Answer from the drawing. Dimensions are ordinates in mm from the lowest x, y and z of the part. A direction names the side the tool comes from. Give positions to 0.01 mm unless a question says otherwise; leave off trailing zeros. Write each loop counter-clockwise with the first axis right and the second up, starting at its lowest first coordinate (ties: lowest second). Pieces come first, ordered by that corner, then holes.
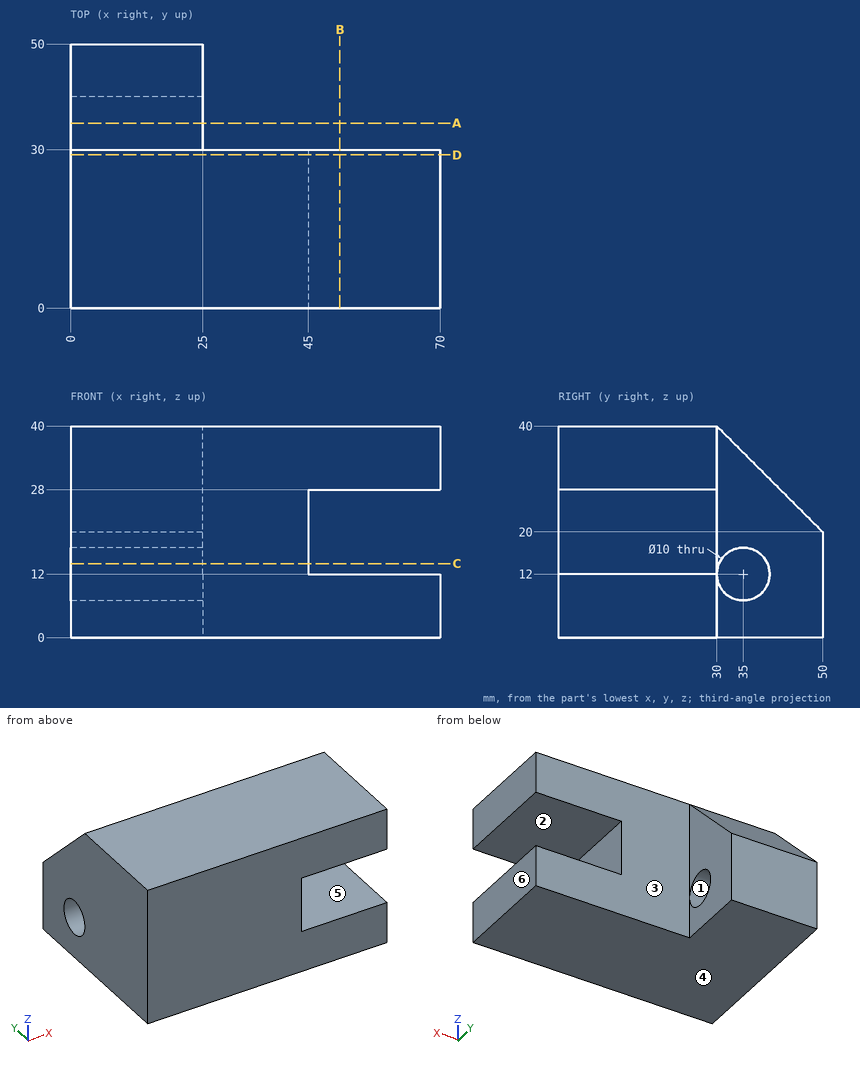
Item 1: Determine the mould class of the marked faces 4, 5 and 6 for opening direction Z: pulls with the +Z half, pulls with the -Z half, needs draft (parallel to the pull), parting line crosses it, or undercut.
Conclusion:
face 4: pulls with the -Z half
face 5: undercut
face 6: needs draft
Item 2: Which of the six approach directions +Z, -Z, +X, -X, +Y, -Y give full straight-line access (tool end or side, diameter ignored) to the marked faces 1, 2 and 3?
Conclusion:
face 1: +X, -X
face 2: +X, +Y, -Y
face 3: +Z, -Z, +X, +Y
Item 3: A cutting plane is placed at D-D, the plane y = 29. Give the vertices of the cut face in (x, z), plus the area to 3 significant figures.
Conclusion:
outline: (0, 0) - (70, 0) - (70, 12) - (45, 12) - (45, 28) - (70, 28) - (70, 40) - (0, 40) - close
area: 2,400 mm2
Item 4: Each of these flat-tipped pins is pushed along its axis until it touches: P1, Ø10, axis at y = 36.5, z = 25.5, coming from the +X side; P2, Ø5, axis at y = 8, z = 23.5, coming from the +X side; P3, Ø5, axis at x = 23.5, z = 35, coming from the +Y side. Where does it stop, or does it pass through?
Conclusion:
P1: stops at x = 25
P2: stops at x = 45
P3: stops at y = 37.5
Item 5: A cutting plane is placed at A-A, the plane y = 35. Give the vertices of the cut face in (x, z).
Conclusion:
outline: (0, 0) - (25, 0) - (25, 7) - (0, 7) - close; (0, 17) - (25, 17) - (25, 35) - (0, 35) - close
Item 6: Consider probe 1 along Z at (x, y) = (57, 22); probe 2 along X at (y, z) = (16, 27); probe 3 along Y at (x, z) = (62.5, 29). Determine where each line is inside the solid, lowest interval first.
Conclusion:
probe 1: z = 0 to 12, 28 to 40
probe 2: x = 0 to 45
probe 3: y = 0 to 30
Item 7: A cutting plane is placed at B-B, the plane x = 51. Give the vertices of the cut face in (y, z), plus the area to 3 significant figures.
Conclusion:
outline: (0, 0) - (30, 0) - (30, 12) - (0, 12) - close; (0, 28) - (30, 28) - (30, 40) - (0, 40) - close
area: 720 mm2
Item 8: A cutting plane is placed at C-C, the plane z = 14. Give the vertices of the cut face in (x, y), plus the area to 3 significant figures.
Conclusion:
outline: (0, 0) - (45, 0) - (45, 30) - (25, 30) - (25, 30.42) - (0, 30.42) - close; (0, 39.58) - (25, 39.58) - (25, 50) - (0, 50) - close
area: 1,620 mm2
